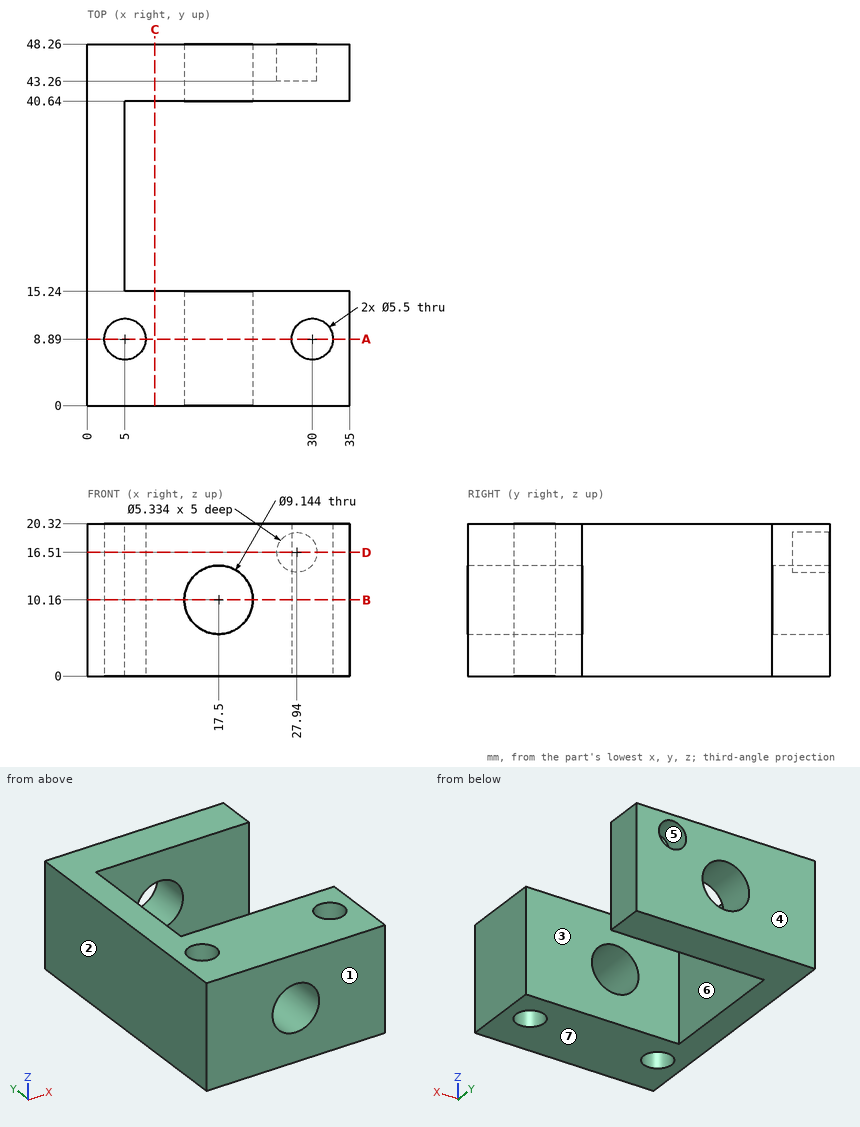
For this review, use the dimensioned drawing (mm, ordinates from the lowest corner) and the shaded views. A direction names the side the tool comes from. Coordinates: 2 decimals unless noted, no trailing zeros. Loops run counter-clockwise (first coordinate to the right, second up) from the corner with the lowest first, then second, coordinate; pieces in that order, holes last. Notation, with made-up numbers: (-13.5, -21.5) -> (11.5, -21.5) arc R6 cw to (11.5, -10.5) -> close; hole circle Ø8 at (54, 7.5). An arc over 180 degrees is marked (long way). Use a Markdown table: item, result. Add a question column.
Item 1: Machinability: for the marked faces 5, 6 and 7, which of the approach directions +Z, -Z, +X, -X, +Y, -Y give a long, thin tool a straight path to every point of the face, cutting with its end or side? Answer none if there is none.
Item 2: We need section B-B, the plane z = 10.16. Write out the cut boundary in (x, y), and give its area (3 significant figures).
Item 3: We need section C-C, the plane x = 9. Write out the cut boundary in (y, z).
Item 4: The part is to be moulded in two halves that separate along Y. For the marked faces 1, 2, 3 and 4, say which applies: +Y half, -Y half, draft (parallel to the pull), parting line (faces both ways), or undercut.
Item 5: We need section D-D, the plane z = 16.51. Write out the cut boundary in (x, y), and give its area (3 significant figures).
Item 6: We need section A-A, the plane y = 8.89. Write out the cut boundary in (x, z), and give its area (3 significant figures).
Item 7: Clearance check with flat-ended pins moving along their axes: P1, Ø6, axis at x = 29, y = 7.5, coming from the -Z side; P2, Ø10, axis at y = 32, z = 6.5, coming from the +X side. State where each tip first meets the part, or that it passes through.
Item 8: Wall thickness on L1, parallel to Y at x = 30, z = 12.5; L2, parallel to Y at x = 22.5, z = 1.5; L3, parallel to Z at x = 17.5, y = 43: over which ranges is each line inside the solid? List them lowest first. Write a range as from..to.
Numbers:
| question | item | result |
|---|---|---|
| 1 | face 5 | +Y |
| 1 | face 6 | +Z, -Z, +X |
| 1 | face 7 | -Z, +X, -X, +Y, -Y |
| 2 | outline | (0, 0) -> (12.93, 0) -> (12.93, 15.24) -> (5, 15.24) -> (5, 40.64) -> (12.93, 40.64) -> (12.93, 48.26) -> (0, 48.26) -> close; (22.07, 0) -> (35, 0) -> (35, 15.24) -> (22.07, 15.24) -> close; (22.07, 40.64) -> (35, 40.64) -> (35, 48.26) -> (22.07, 48.26) -> close; hole circle Ø5.5 at (5, 8.89); hole circle Ø5.5 at (30, 8.89) |
| 2 | area | 671 mm^2 |
| 3 | outline | (0, 0) -> (15.24, 0) -> (15.24, 20.32) -> (0, 20.32) -> close; (40.64, 0) -> (48.26, 0) -> (48.26, 20.32) -> (40.64, 20.32) -> close |
| 4 | face 1 | -Y half |
| 4 | face 2 | draft |
| 4 | face 3 | undercut |
| 4 | face 4 | +Y half |
| 5 | outline | (0, 0) -> (35, 0) -> (35, 15.24) -> (5, 15.24) -> (5, 40.64) -> (35, 40.64) -> (35, 48.26) -> (30.61, 48.26) -> (30.61, 43.26) -> (25.27, 43.26) -> (25.27, 48.26) -> (0, 48.26) -> close; hole circle Ø5.5 at (5, 8.89); hole circle Ø5.5 at (30, 8.89) |
| 5 | area | 853 mm^2 |
| 6 | outline | (0, 0) -> (2.25, 0) -> (2.25, 20.32) -> (0, 20.32) -> close; (7.75, 0) -> (27.25, 0) -> (27.25, 20.32) -> (7.75, 20.32) -> close; (32.75, 0) -> (35, 0) -> (35, 20.32) -> (32.75, 20.32) -> close; hole circle Ø9.14 at (17.5, 10.16) |
| 6 | area | 422 mm^2 |
| 7 | P1 | stops at z = 0 |
| 7 | P2 | stops at x = 5 |
| 8 | L1 | y = 0..6.14, 11.64..15.24, 40.64..48.26 |
| 8 | L2 | y = 0..15.24, 40.64..48.26 |
| 8 | L3 | z = 0..5.59, 14.73..20.32 |
